Geometry: final body of the model. Coordinates: model frame, mm. A direction names the side the tool comes from. Coordinates: 2 decimals unless noted, no trailing zeros. Write each loop counter-clockwise with the first axis right and the second up, starting at its lowest first coordinate (ties: lowest second). Pieces come first, ordered by that corner, then holes. Notation, with made-up numbers: (50, 0) - (101, 0) arc R22 ccw to (101, 38) - close; hole circle Ø3 at (-17.75, 19.25). An arc over 180 degrees is marked (long way). Put each result on its own line as item: value.
```python
from build123d import *

# Parameters (mm, degrees)
F0_W     = 56
F0_H     = 16
F1_DEPTH = 25
F2_W     = 16
F2_H     = 16
F3_DEPTH = 12.5
F4_R     = 4
F7_DEPTH = 25
F8_DEPTH = 25
F9_SIZE  = 0.2


with BuildPart() as f1:
    # F0 (on Top) → F1 (new body)
    with BuildSketch(Plane.XY):
        with Locations((-3.4085810184, -0.5300787467)):
            Rectangle(F0_W, F0_H)
    extrude(amount=F1_DEPTH)

    # F2 (on face) → F3 (cut)
    with BuildSketch(Plane.XY.offset(25)):
        with Locations((2.5914189816, -0.5300787467)):
            Rectangle(F2_W, F2_H)
    extrude(amount=-F3_DEPTH, mode=Mode.SUBTRACT)

    # F4
    f4_edges = [f1.edges().sort_by_distance(p)[0] for p in [
        (10.591419, -0.530079, 12.5),
        (-5.408581, -0.530079, 12.5),
    ]]
    fillet(f4_edges, radius=F4_R)

    # F6 (on face) → F7 (cut)
    with BuildSketch(Plane.XZ.offset(8.5300787467)):
        Polygon((24.5914189816, 25), (19.0914189816, 25), (24.5914189816, 7.0707142143), align=None)
        Polygon((24.5914189816, 0), (24.5914189816, 3.5707142143), (21.0914189816, 0), align=None)
    extrude(amount=-F7_DEPTH, mode=Mode.SUBTRACT)

    # F5 (on face) → F8 (cut)
    with BuildSketch(Plane.XY.offset(25)):
        Polygon((19.0914189816, 7.4699212533), (12.5914189816, 7.4699212533), (19.0914189816, 4.4699212533), align=None)
        Polygon((19.0914189816, -5.5300787467), (12.5914189816, -8.5300787467), (19.0914189816, -8.5300787467), align=None)
        Polygon((19.0914189816, 7.4699212533), (19.0914189816, 4.4699212533), (24.5914189816, 1.9314597149), (24.5914189816, 7.4699212533), align=None)
        Polygon((24.5914189816, -8.5300787467), (24.5914189816, -2.9916172082), (19.0914189816, -5.5300787467), (19.0914189816, -8.5300787467), align=None)
    extrude(amount=-F8_DEPTH, mode=Mode.SUBTRACT)

    # F9
    f9_edges = [f1.edges().sort_by_distance(p)[0] for p in [
        (-18.408581, -8.530079, 25),
        (-18.408581, 7.469921, 25),
        (11.591419, 7.469921, 25),
        (11.591419, -8.530079, 25),
        (-9.408581, -8.530079, 0),
        (-9.408581, 7.469921, 0),
    ]]
    chamfer(f9_edges, length=F9_SIZE)


solid = f1.part
```
1. Set-up query: faces 4 (the flat face through (3, 0, 12.5)), 5 (the flat face through (21.192, -0.6, 18.153)). Return all of +Z, -Z, +X, -X, +Y, -Y with unobstructed straight access to the full face (end or side cutting, diameter ignored); none if empty.
Answer below:
face 4: +Z, +Y, -Y
face 5: +Z, +X, +Y, -Y
2. Pin query (flat end, axial travel): pin 1 Ø8 at (y, z) = (1.5, 15) entering from +X; pin 2 Ø6.5 at (x, y) = (1, 2) entering from +Z; pin 3 Ø9.5 at (y, z) = (-4, 19.5) entering from +X. Return the tip coordinate at first contact, or that it passes through.
Answer below:
pin 1: stops at x = 23.39
pin 2: stops at z = 12.59
pin 3: stops at x = 22.24
3. Section query A-A (y = -2). Return loops of the section in (x, z).
Answer below:
outline: (-31.41, 0) - (21.09, 0) - (24.59, 3.57) - (24.59, 7.07) - (19.09, 25) - (10.59, 25) - (10.59, 16.5) arc R4 cw to (6.59, 12.5) - (-1.41, 12.5) arc R4 cw to (-5.41, 16.5) - (-5.41, 25) - (-31.41, 25) - close
4. Section query C-C (z = 14.5). Return loops of the section in (x, y).
Answer below:
outline: (-31.41, -8.53) - (-4.87, -8.53) - (-4.87, 7.47) - (-31.41, 7.47) - close; (10.06, -8.53) - (12.59, -8.53) - (22.31, -4.04) - (22.31, 2.98) - (12.59, 7.47) - (10.06, 7.47) - close
5. Mould query, pull axis X, two halves, no side actions, for faces 1 (the flat face through (-6, 0, 0)), 2 (the flat face through (10.591, -1, 21)), 3 (the flat face through (24.591, -1, 5)). Classes: +X half, -X half, draft (parallel to the pull), parting line (faces both ways), or undercut.
Answer below:
face 1: draft
face 2: undercut
face 3: +X half
6. Ray query, probe 1 along X at (y, z) = (-3.75, 23.25); probe 2 along X at (y, z) = (-0.5, 13.5); probe 3 along Z at (x, y) = (4.5, -5.5). Return the intervals inside material, ascending. Write a range as from..to.
Answer below:
probe 1: x = -31.41..-5.41, 10.59..19.63
probe 2: x = -31.41..-4.05, 9.24..22.62
probe 3: z = 0..12.5
7. Section query D-D (x = -2). Return loops of the section in (y, z).
Answer below:
outline: (-8.53, 0.2) - (-8.33, 0) - (7.27, 0) - (7.47, 0.2) - (7.47, 12.54) - (-8.53, 12.54) - close
8. Section query B-B (z = 6.5). Return loops of the section in (x, y), then the cut area to 3 significant figures.
Answer below:
outline: (-31.41, -8.53) - (12.59, -8.53) - (24.59, -2.99) - (24.59, 1.93) - (12.59, 7.47) - (-31.41, 7.47) - close
area: 830 mm²
